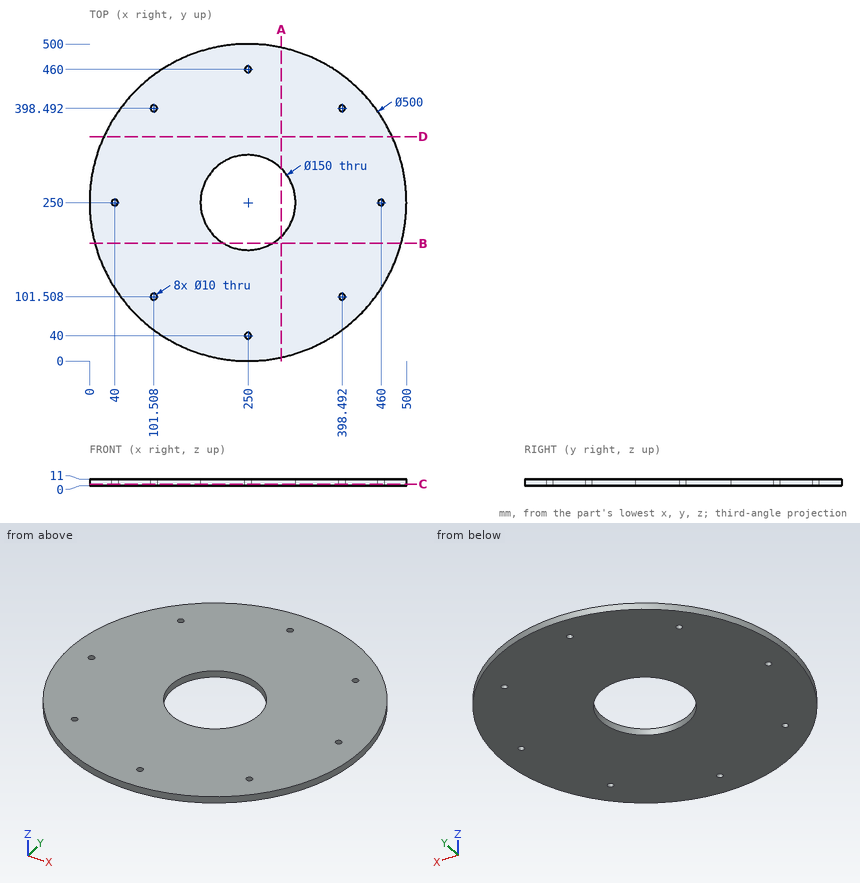
Answer from the drawing. Dimensions are ordinates in mm from the lowest x, y and z of the part. Give positions to 0.01 mm unless a question says otherwise; leave off trailing zeros. Order: outer loops, then holes, each group sorted by start corner. A loop starts at its lowest first (then second) coordinate and runs counter-clockwise, first axis right, second up.
Item 1: The part is cut by section A-A, the plane x = 302.5. Give the vertices of the cut face in (y, z) (1 decimal).
From the geometry:
outline: (5.6, 0) - (196.4, 0) - (196.4, 11) - (5.6, 11) - close; (303.6, 0) - (494.4, 0) - (494.4, 11) - (303.6, 11) - close
Item 2: Given pin 1 Ø9 at (x, y) = (101.51, 398.49) entering from +Z; pin 2 Ø5 at (y, z) = (329, 5.5) entering from +X; pin 3 Ø4 at (x, z) = (392, 3) entering from +Y; pin 4 Ø13 at (x, y) = (40, 250) entering from +Z, each flat-ended and moving along its own axis, determine where each tip first touches the part or whether it passes through.
From the geometry:
pin 1: passes through
pin 2: stops at x = 488.01
pin 3: stops at y = 457.12
pin 4: stops at z = 11
Item 3: Find the intervals of material crossed by probe 1 along Y at (x, z) = (250, 5.5); probe 2 along Y at (x, z) = (234, 7.5); probe 3 along X at (y, z) = (192.5, 5) (1 decimal), in increasing order.
From the geometry:
probe 1: y = 0 to 35, 45 to 175, 325 to 455, 465 to 500
probe 2: y = 0.51 to 176.73, 323.27 to 499.49
probe 3: x = 6.7 to 201.8, 298.2 to 493.3
Item 4: The part is cut by section C-C, the plane z = 2.75. Count the separate pieces of the cut face and the enclosed holes in it, and give its area (3 significant figures).
From the geometry:
separate pieces: 1
enclosed holes: 9
area: 178,000 mm2
Item 5: The part is cut by section D-D, the plane y = 354. Give the vertices of the cut face in (x, z), and give its area (3 significant figures).
From the geometry:
outline: (22.66, 0) - (477.34, 0) - (477.34, 11) - (22.66, 11) - close
area: 5,000 mm2
Item 6: The part is cut by section B-B, the plane y = 185.5. Give the vertices of the cut face in (x, z), and give its area (3 significant figures).
From the geometry:
outline: (8.46, 0) - (211.73, 0) - (211.73, 11) - (8.46, 11) - close; (288.27, 0) - (491.54, 0) - (491.54, 11) - (288.27, 11) - close
area: 4,470 mm2
